Answer from the drawing. Dimensions are ordinates in mm from the lowest x, y and z of the part. Give positions to 0.01 mm unless a question says otherwise; leave off trailing zeros. Order: outer loops, then holes, each group sorted by start corner. A loop starts at its lowest first (then second) coordinate and runs counter-clockwise, first axis right, second up.
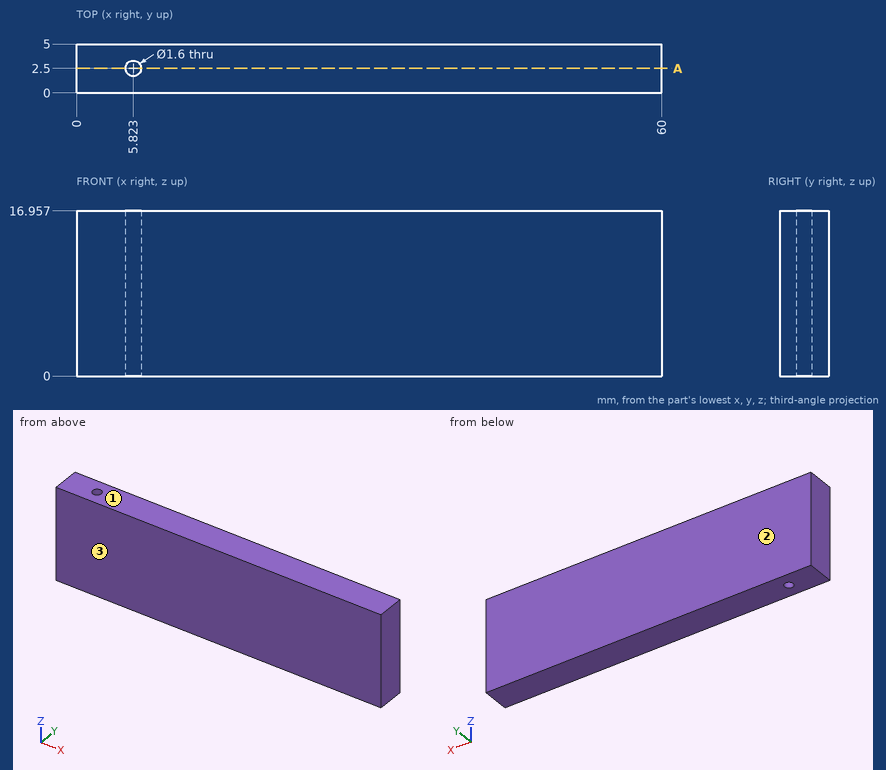
1) The part is cut by section A-A on y = 2.5. Determine the outline of the cut face in (x, z).
Final values:
outline: (0, 0) - (5.02, 0) - (5.02, 16.96) - (0, 16.96) - close; (6.62, 0) - (60, 0) - (60, 16.96) - (6.62, 16.96) - close
2) Consider L1, parallel to X at y = 2.45, z = 5 (1 decimal); L2, parallel to X at y = 3, z = 4.5. Determine where each line is inside the solid, lowest interval first.
Final values:
L1: x = 0 to 5, 6.6 to 60
L2: x = 0 to 5.2, 6.45 to 60
3) For a pull along Y with two mould halves and no side action, classify the marked faces 1, 2 and 3 as released by +Y, released by -Y, zero draft, split by the parting line, or undercut.
Final values:
face 1: zero draft
face 2: released by +Y
face 3: released by -Y
